Could you check a few things on this model? Use its own coordinates, in mm. Face numbers are marked on the shaded views. A direction names the side the tool comes from. Give positions to 0.01 mm unless a question says otherwise; leave off trailing zeros. Order: outer loops, then holes, each group sorted by start corner. A loop starts at its lowest first (then second) coordinate and runs counter-clockwise, first axis right, second up. Notation, with made-up numbers: (55, 85) -> (93, 85) arc R13 cw to (93, 101) -> close; hole circle Ø5 at (-25, -1). An arc over 180 degrees is marked (long way). One line per item, written item: value.
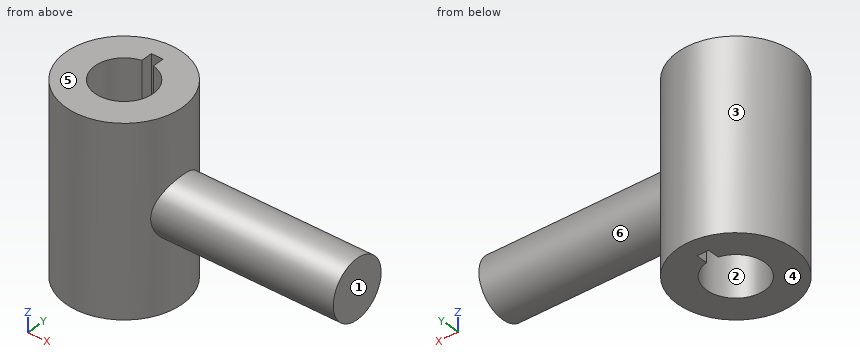
```python
from build123d import *

# Parameters (mm, degrees)
SKETCH1_R                = 6.35
BOSS_EXTRUDE1_DEPTH      = 10.16
BOSS_EXTRUDE2_REACH      = 35.935
BOSS_EXTRUDE2_END_RADIUS = 6.35
SKETCH2_R                = 3.175


with BuildPart() as part:
    # Sketch1 → Boss-Extrude1 (new, symmetric)
    with BuildSketch(Plane.XY):
        Circle(SKETCH1_R)
        with BuildLine():
            Line((-0.635, 3.110851973), (-0.635, 4.380851973))
            Line((-0.635, 4.380851973), (0.635, 4.380851973))
            Line((0.635, 4.380851973), (0.635, 3.110851973))
            ThreePointArc((0.635, 3.110851973), (0, -3.175), (-0.635, 3.110851973))
        make_face(mode=Mode.SUBTRACT)
    extrude(amount=BOSS_EXTRUDE1_DEPTH, both=True)

    # Boss-Extrude2: up to this cylinder (the profile starts outside it)
    boss_extrude2_end = Plane(origin=(0, 0, 0), z_dir=(0, 0, -1)) * Cylinder(BOSS_EXTRUDE2_END_RADIUS, 85.57, mode=Mode.PRIVATE)
    # Sketch2 → Boss-Extrude2 (add, up to the surface)
    with BuildSketch(Plane(origin=(25.4, 0, 0), x_dir=(0, 0, -1), z_dir=(1, 0, 0)), mode=Mode.PRIVATE) as boss_extrude2_sk1:
        Circle(SKETCH2_R)
    boss_extrude2_tool1 = extrude(boss_extrude2_sk1.sketch, amount=-BOSS_EXTRUDE2_REACH, mode=Mode.PRIVATE) - boss_extrude2_end
    add(boss_extrude2_tool1.solids().sort_by_distance((25.4, 0, 0))[0])


solid = part.part
```
1) Suppose I cut it at A-A, the plane x = 0. Write out the boundary of the cut face in (y, z) (3 decimals).
Answer below:
outline: (-6.35, -10.16) -> (-3.175, -10.16) -> (-3.175, 10.16) -> (-6.35, 10.16) -> close; (4.381, -10.16) -> (6.35, -10.16) -> (6.35, 10.16) -> (4.381, 10.16) -> close
2) We'd pull the mould along X, two halves only. Please class the marked faces 1, 2, 3 and 4: +X half, -X half, draft (parallel to the pull), parting line (faces both ways), or undercut.
Answer below:
face 1: +X half
face 2: undercut
face 3: parting line
face 4: draft
3) If I drill on line 1 along Y through (x, z) = (-1.5, -2.25); line 2 along X through (y, z) = (0.75, -1.25); line 3 along X through (y, z) = (2.25, -8.25), over which ranges is the centre line in solid material (lowest first)?
Answer below:
line 1: y = -6.17 to -2.8, 2.8 to 6.17
line 2: x = -6.31 to -3.09, 3.09 to 25.4
line 3: x = -5.94 to -2.24, 2.24 to 5.94
4) Suppose I cut it at C-C, the plane z = 0. Write out the boundary of the cut face in (x, y) (3 decimals), then the cut area to 3 significant figures.
Answer below:
outline: (5.499, -3.175) -> (25.4, -3.175) -> (25.4, 3.175) -> (5.499, 3.175) arc R6.35 ccw (long way) to start; hole (-0.635, 3.111) arc R3.175 ccw (long way) to (0.635, 3.111) -> (0.635, 4.381) -> (-0.635, 4.381) -> close
area: 216 mm2
5) Suppose I cut it at B-B, the plane y = 0. Write out the boundary of the cut face in (x, z) (3 decimals).
Answer below:
outline: (-6.35, -10.16) -> (-3.175, -10.16) -> (-3.175, 10.16) -> (-6.35, 10.16) -> close; (3.175, -10.16) -> (6.35, -10.16) -> (6.35, -3.175) -> (25.4, -3.175) -> (25.4, 3.175) -> (6.35, 3.175) -> (6.35, 10.16) -> (3.175, 10.16) -> close
6) For the marked faces 5 and 6, which set-ups out of +Z, -Z, +X, -X, +Y, -Y let a thin tool reach every point of the face, with its end or its side?
Answer below:
face 5: +Z, +X, -X, +Y, -Y
face 6: +X
7) For P1, Ø12, axis at x = 15.5, z = -5, coming from the -Y side (3 decimals); P2, Ø0.6, axis at y = 4, z = -3.5, coming from the -X side; P3, Ø1.4, axis at y = 4, z = 0.5, coming from the +X side, each with a flat end and sliding along its axis, tell me the tip position at first contact or that it passes through.
Answer below:
P1: stops at y = -3.175
P2: stops at x = -5.16
P3: stops at x = 5.43
8) Suppose I cut it at D-D, the plane z = -8.5. Write out the boundary of the cut face in (x, y) (3 decimals), then the cut area to 3 significant figures.
Answer below:
outline: circle Ø12.7 at (0, 0); hole (-0.635, 3.111) arc R3.175 ccw (long way) to (0.635, 3.111) -> (0.635, 4.381) -> (-0.635, 4.381) -> close
area: 93.4 mm2
